Source: three-view drawing plus pictorial views. Frame: mm from the lowest corner of the part. Give positions to 0.01 mm unless a question says otherwise; leave off trailing zeros. Loops run counter-clockwise (first coordinate to the right, second up) from the corner with the lowest first, then second, coordinate; pieces in that order, holes last. Notation, with made-up numbers: (3.25, -14.5) -> (9.25, -14.5) arc R10 cw to (9.25, 0.5) -> close; hole circle Ø4 at (42, 49). An arc over 180 degrees is marked (long way). Answer as a JSON object with one key per item and string values. Group by question number.
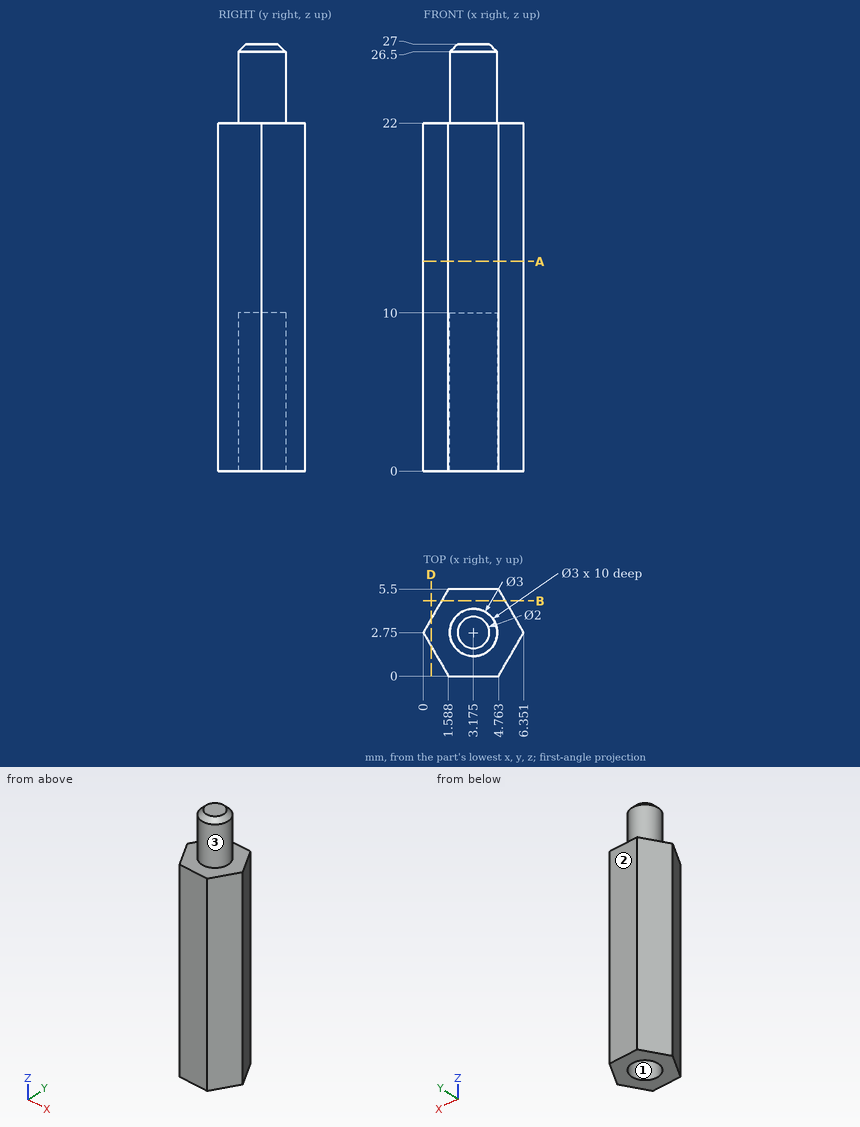
(1) Section query B-B on y = 4.75. Return the cut outline in (x, z) (1 decimal).
(2) Mould query, pull axis Y, two halves, no side actions, for the marked faces 1, 2 and 3. Classes: pulls with the +Y half, pulls with the -Y half, needs draft (parallel to the pull), parting line crosses it, or undercut.
(3) Material intervals for line 1 (Z direction, x = 1.5, y = 4.7); line 2 (Y direction, x = 2, z = 7); line 3 (X direction, y = 1.4, z = 5.25) (1 decimal), sorted ascending. Write a range as from..to.
(4) Section query D-D on x = 0.5. Return the cut outline in (y, z), plus the area to 3 significant figures.
(5) Section query A-A on z = 13.25. Return the cut outline in (x, y), plus the area to 3 significant figures.
Result:
{
 "1": {"outline": "(1.2, 0) -> (5.2, 0) -> (5.2, 22) -> (1.2, 22) -> close"},
 "2": {"face 1": "undercut", "face 2": "pulls with the +Y half", "face 3": "parting line crosses it"},
 "3": {"line 1": "0..22", "line 2": "0..1.82, 3.68..5.5", "line 3": "0.8..2.5, 3.8..5.6"},
 "4": {"outline": "(1.88, 0) -> (3.62, 0) -> (3.62, 22) -> (1.88, 22) -> close", "area": "38.1 mm²"},
 "5": {"outline": "(0, 2.75) -> (1.59, 0) -> (4.76, 0) -> (6.35, 2.75) -> (4.76, 5.5) -> (1.59, 5.5) -> close", "area": "26.2 mm²"}
}
